```python
from build123d import *

# Parameters (mm, degrees)
EXTRUDE_THIN2_DEPTH     = 140
SKETCH11_W              = 166
SKETCH11_H              = 5
BOSS_EXTRUDE3_DEPTH     = 2.6416
CUT_EXTRUDE6_DEPTH      = 255.903903462
CUT_EXTRUDE6_DEPTH_BACK = 255.903903462
SKETCH13_W              = 40
SKETCH13_H              = 5
CUT_EXTRUDE7_DEPTH      = 258.480096318
SKETCH19_W              = 4
SKETCH19_H              = 130
CUT_EXTRUDE9_DEPTH      = 10
SKETCH20_W              = 4
SKETCH20_H              = 130
CUT_EXTRUDE10_DEPTH     = 10
SKETCH21_W              = 6
SKETCH21_H              = 77
BOSS_EXTRUDE4_DEPTH     = 110


with BuildPart() as part:
    # Sketch2 → Extrude-Thin2 (new body)
    with BuildSketch(Plane.XY):
        Polygon((0, 120), (0, 0), (186, 0), (186, 120), (176, 120), (176, 10), (10, 10), (10, 120), align=None)
    extrude(amount=EXTRUDE_THIN2_DEPTH)

    # Sketch11 → Boss-Extrude3 (add)
    with BuildSketch(Plane(origin=(0, 10, 0), x_dir=(1, 0, 0), z_dir=(0, 1, 0))):
        with Locations((93, -6.5)):
            Rectangle(SKETCH11_W, SKETCH11_H)
    extrude(amount=BOSS_EXTRUDE3_DEPTH)

    # Sketch13 → Cut-Extrude6 (cut, two sides: drawn at the far end of the back side and taken through both)
    with BuildSketch(Plane(origin=(10, 0, 0), x_dir=(0, 0, -1), z_dir=(1, 0, 0)).offset(-CUT_EXTRUDE6_DEPTH_BACK)):
        with Locations((-113.795011338, 89.551599899)):
            Rectangle(SKETCH13_W, SKETCH13_H)
    extrude(amount=CUT_EXTRUDE6_DEPTH + CUT_EXTRUDE6_DEPTH_BACK, mode=Mode.SUBTRACT)

    # Sketch14 → Cut-Extrude7 (cut, through all)
    with BuildSketch(Plane(origin=(0, 10, 0), x_dir=(1, 0, 0), z_dir=(0, 1, 0))):
        with BuildLine():
            Line((176, -140), (10, -140))
            ThreePointArc((10, -140), (93, -110), (176, -140))
        make_face()
    extrude(amount=-CUT_EXTRUDE7_DEPTH, mode=Mode.SUBTRACT)

    # Sketch19 → Cut-Extrude9 (cut)
    with BuildSketch(Plane(origin=(0, 120, 0), x_dir=(1, 0, 0), z_dir=(0, 1, 0))):
        with Locations((5, -70)):
            Rectangle(SKETCH19_W, SKETCH19_H)
    extrude(amount=-CUT_EXTRUDE9_DEPTH, mode=Mode.SUBTRACT)

    # Sketch20 → Cut-Extrude10 (cut)
    with BuildSketch(Plane(origin=(0, 120, 0), x_dir=(1, 0, 0), z_dir=(0, 1, 0))):
        with Locations((181, -70)):
            Rectangle(SKETCH20_W, SKETCH20_H)
    extrude(amount=-CUT_EXTRUDE10_DEPTH, mode=Mode.SUBTRACT)

    # Sketch21 → Boss-Extrude4 (add, through all)
    with BuildSketch(Plane(origin=(0, 10, 0), x_dir=(1, 0, 0), z_dir=(0, 1, 0))):
        with Locations((93, -49.5)):
            Rectangle(SKETCH21_W, SKETCH21_H)
    extrude(amount=BOSS_EXTRUDE4_DEPTH)


solid = part.part
```
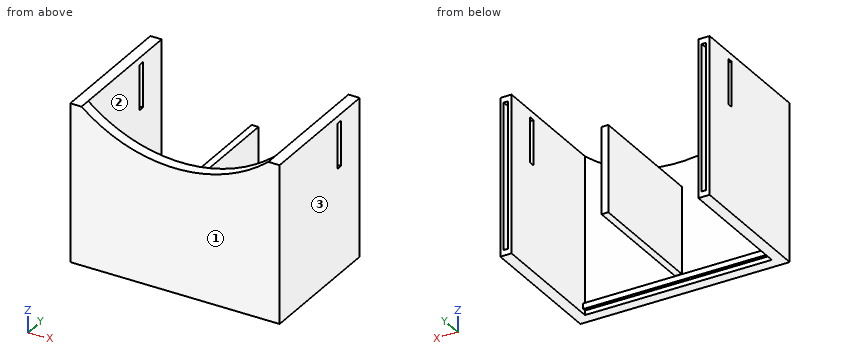
The model under review builds one solid part; all positions refer to its coordinate system, in mm. Face numbers are marked on the shaded views. Round coordinates to 2 decimals unless told otherwise and drop trailing zeros. Write each loop counter-clockwise with the first axis right and the second up, starting at its lowest first coordinate (ties: lowest second). Pieces come first, ordered by that corner, then holes.
(1) We need section B-B on z = 123.5. Give the boundary of the cut face in (x, y).
(2) We need section A-A on y = 41. Give the boundary of the cut face in (x, z), and give its area (3 significant figures).
(3) We need section C-C on z = 58.5. Give the boundary of the cut face in (x, y).
(4) Insertion check: pin 1 (3 mm diameter, centred on x = 110, z = 82, fed in from +Y); pin 2 (2.5 mm diameter, centred on x = 124.5, z = 6.5, fed in from +Y); pin 3 (3 mm diameter, centred on x = 93, y = 88, fed in from +Z). Each pin has a flat end and moves straight along its axis. Give the tip position at first contact, or say it passes through.
(5) We need section D-D on x = 38.5. Give the boundary of the cut face in (y, z), and give its area (3 significant figures).
(6) Wall thickness on L1, parallel to X at y = 53, z = 64.5; L2, parallel to X at y = 27.5, z = 95; L3, parallel to Y at x = 55.5, z = 15: over which ranges is each line inside the solid? List them lowest first.
(7) Mouldability with a two-part tool opening along X and no side actions: class the marked faces 1, 2 and 3 as +X half, -X half, draft (parallel to the pull), parting line (faces both ways), or undercut.
Findings below:
1. outline: (0, 0) - (35.36, 0) - (35.36, 10) - (10, 10) - (10, 87.05) - (0, 87.05) - close; (0, 92.05) - (10, 92.05) - (10, 120) - (7, 120) - (7, 110) - (3, 110) - (3, 120) - (0, 120) - close; (150.64, 0) - (186, 0) - (186, 87.05) - (176, 87.05) - (176, 10) - (150.64, 10) - close; (176, 92.05) - (186, 92.05) - (186, 120) - (183, 120) - (183, 110) - (179, 110) - (179, 120) - (176, 120) - close
2. outline: (0, 0) - (10, 0) - (10, 140) - (0, 140) - close; (90, 11) - (96, 11) - (96, 88) - (90, 88) - close; (176, 0) - (186, 0) - (186, 140) - (176, 140) - close
2. area: 3,260 mm2
3. outline: (0, 0) - (186, 0) - (186, 120) - (183, 120) - (183, 110) - (179, 110) - (179, 120) - (176, 120) - (176, 10) - (96, 10) - (96, 120) - (90, 120) - (90, 10) - (10, 10) - (10, 120) - (7, 120) - (7, 110) - (3, 110) - (3, 120) - (0, 120) - close
4. pin 1: stops at y = 10
4. pin 2: stops at y = 12.64
4. pin 3: stops at z = 88
5. outline: (0, 0) - (10, 0) - (10, 4) - (12.64, 4) - (12.64, 9) - (10, 9) - (10, 121.99) - (0, 121.99) - close
5. area: 1,230 mm2
6. L1: x = 0 to 10, 90 to 96, 176 to 186
6. L2: x = 0 to 10, 176 to 186
6. L3: y = 0 to 10
7. face 1: draft
7. face 2: undercut
7. face 3: +X half
